```python
from build123d import *

# Parameters (mm, degrees)
SKETCH_1_R      = 3
EXTRUDE_1_DEPTH = 3
FILLET_1_R      = 1


with BuildPart() as part:
    # 草图1 → 凸台-拉伸1 (new body)
    with BuildSketch(Plane(origin=(0, 0, 0), x_dir=(0, 0, -1), z_dir=(1, 0, 0))):
        with BuildLine():
            Line((-15, 7), (15, 7))
            ThreePointArc((15, 7), (22, 0), (15, -7))
            Line((15, -7), (-15, -7))
            ThreePointArc((-15, -7), (-22, 0), (-15, 7))
        make_face()
        with Locations((-15, 0)):
            Circle(SKETCH_1_R, mode=Mode.SUBTRACT)
        with Locations((15, 0)):
            Circle(SKETCH_1_R, mode=Mode.SUBTRACT)
    extrude(amount=EXTRUDE_1_DEPTH)

    # 圆角1
    fillet_1_edges = [part.edges().sort_by_distance(p)[0] for p in [
        (3, 0, -22),
        (3, 7, 0),
        (3, 0, 22),
        (0, 7, 0),
        (0, 0, -22),
        (0, -7, 0),
        (0, 0, 22),
        (3, -7, 0),
    ]]
    fillet(fillet_1_edges, radius=FILLET_1_R)


solid = part.part
```
Here's how the part is built. I have some questions about the finished solid (model axes, mm). Coordinates: 2 decimals unless noted, no trailing zeros. Loops run counter-clockwise (first coordinate to the right, second up) from the corner with the lowest first, then second, coordinate; pieces in that order, holes last. Notation, with made-up numbers: M -5,-2.5 L 41,-2.5 A35 cw 41,30.5 Z; hole C 81.5,-13 d6. An arc over 180 degrees is marked long. One line per item, written item: value.
1. Thinking about a two-plate mould opening in Y: for faces 1 (the cylindrical face through (1, 0, 18)), 2 (the cylindrical face through (0.301, 6.715, -0.21)), 3 (the cylindrical face through (0.301, -6.715, 0.21)), which applies, +Y half, -Y half, draft (parallel to the pull), parting line (faces both ways), or undercut?
Geometry says:
face 1: undercut
face 2: +Y half
face 3: -Y half
2. Imagine slicing it at B-B (x = 1.55). List the corners of the cut face in (y, z) for me.
Geometry says:
outline: M -7,-15 A7 ccw 7,-15 L 7,15 A7 ccw -7,15 Z; hole C 0,-15 d6; hole C 0,15 d6
3. Imagine slicing it at A-A (y = 0). List the corners of the cut face in (x, z) for me.
Geometry says:
outline: M 0,-21 A1 ccw 1,-22 L 2,-22 A1 ccw 3,-21 L 3,-18 L 0,-18 Z; M 0,-12 L 3,-12 L 3,12 L 0,12 Z; M 0,18 L 3,18 L 3,21 A1 ccw 2,22 L 1,22 A1 ccw 0,21 Z
4. Please list where these lines run through material, in increasing order: probe 1 along Z at (x, y) = (1.8, 1.75); probe 2 along Z at (x, y) = (2, -1); probe 3 along Y at (x, z) = (2.1, -15).
Geometry says:
probe 1: z = -21.78 to -17.44, -12.56 to 12.56, 17.44 to 21.78
probe 2: z = -21.93 to -17.83, -12.17 to 12.17, 17.83 to 21.93
probe 3: y = -6.99 to -3, 3 to 6.99
5. Imagine slicing it at D-D (y = 1.75). State how many separate pieces and enclosed holes the cut face has, and give its area (3 significant figures).
Geometry says:
separate pieces: 3
enclosed holes: 0
area: 101 mm2
6. Will these pins go through, and if not, where does the flat tip stop? pin 1 Ø8 at (y, z) = (0, 15) entering from +X; pin 2 Ø1.5 at (x, z) = (1.5, 16.5) entering from -Y.
Geometry says:
pin 1: stops at x = 3
pin 2: stops at y = -6.96
7. Imagine slicing it at C-C (z = -10). List the corners of the cut face in (x, y) for me.
Geometry says:
outline: M 0,-6 A1 ccw 1,-7 L 2,-7 A1 ccw 3,-6 L 3,6 A1 ccw 2,7 L 1,7 A1 ccw 0,6 Z
